```python
from build123d import *

# Parameters (mm, degrees)
SKETCH4_W                      = 116
SKETCH4_H                      = 116
BOSS_EXTRUDE1_DEPTH            = 10
SKETCH6_R                      = 33.5
CUT_EXTRUDE1_DEPTH             = 83.63171304
BOSS_EXTRUDE3_DEPTH            = 8.4
SKETCH10_W                     = 116
SKETCH10_H                     = 116
BOSS_EXTRUDE5_DEPTH            = 15
SKETCH11_R                     = 4
POSITIONING_HOLE_DEPTH         = 28
SKETCH23_R                     = 4
SNAPPING_HOLE_DEPTH            = 28
SKETCH13_R                     = 34.75
SKETCH13_R_2                   = 33.5
BOSS_EXTRUDE6_DEPTH            = 25
SKETCH24_W                     = 40
SKETCH24_H                     = 8
BOSS_EXTRUDE7_DEPTH            = 150
BOSS_EXTRUDE9_DEPTH            = 40
CUT_EXTRUDE6_DEPTH             = 8
CUT_EXTRUDE6_DIRECTION_2_REACH = 229.876
CUT_EXTRUDE7_REACH             = 225.194
CUT_EXTRUDE9_REACH             = 209.566
SKETCH37_W                     = 25
SKETCH37_H                     = 20
SKETCH12_R                     = 33.5
MAIN_HOLE_DEPTH                = 179.740034687
SKETCH42_R                     = 54
SKETCH42_R_2                   = 51
BOSS_EXTRUDE12_DEPTH           = 150
CHAMFER3_SIZE                  = 5
SKETCH44_W                     = 40.182717611
SKETCH44_H                     = 23
BOSS_EXTRUDE15_DEPTH           = 150
SKETCH41_R                     = 2
BOSS_EXTRUDE11_DEPTH           = 5
CUT_EXTRUDE12_START            = -150
SKETCH45_R                     = 51
CUT_EXTRUDE12_DEPTH            = 150
SKETCH46_R                     = 1
CUT_EXTRUDE13_DEPTH            = 25


with BuildPart() as part:
    # Sketch4 → Boss-Extrude1 (new body)
    with BuildSketch(Plane(origin=(0, 0, 0), x_dir=(1, 0, 0), z_dir=(0, 1, 0))):
        Rectangle(SKETCH4_W, SKETCH4_H)
    extrude(amount=BOSS_EXTRUDE1_DEPTH)

    # Sketch6 → Cut-Extrude1 (cut, through all)
    with BuildSketch(Plane(origin=(0, 10, 0), x_dir=(1, 0, 0), z_dir=(0, 1, 0))):
        with Locations(Location((0, 0, 0), (0, 0, 270))):
            Circle(SKETCH6_R)
    extrude(amount=-CUT_EXTRUDE1_DEPTH, mode=Mode.SUBTRACT)

    # Sketch8 → Boss-Extrude3 (add)
    with BuildSketch(Plane.XZ):
        with BuildLine():
            Line((-58, 58), (-58, -58))
            Line((-58, -58), (22, -58))
            ThreePointArc((22, -58), (-36, 0), (22, 58))
            Line((22, 58), (-58, 58))
        make_face()
    extrude(amount=BOSS_EXTRUDE3_DEPTH)

    # Sketch10 → Boss-Extrude5 (add)
    with BuildSketch(Plane.XZ.offset(8.4)):
        Rectangle(SKETCH10_W, SKETCH10_H)
    extrude(amount=BOSS_EXTRUDE5_DEPTH)

    # Sketch11 → positioning hole (cut)
    with BuildSketch(Plane.XZ.offset(23.4)):
        with Locations(Location((39, 0, 0), (0, 0, 270))):
            Circle(SKETCH11_R)
    extrude(amount=-POSITIONING_HOLE_DEPTH, mode=Mode.SUBTRACT)

    # Sketch23 → snapping hole (cut)
    with BuildSketch(Plane.XZ.offset(23.4)):
        with Locations(Location((38.947036647, 20, 0), (0, 0, 270))):
            Circle(SKETCH23_R)
    extrude(amount=-SNAPPING_HOLE_DEPTH, mode=Mode.SUBTRACT)

    # Sketch13 → Boss-Extrude6 (add)
    with BuildSketch(Plane.XZ.offset(23.4)):
        with Locations(Location((0, 0, 0), (0, 0, 270))):
            Circle(SKETCH13_R)
        with Locations(Location((0, 0, 0), (0, 0, 90))):
            Circle(SKETCH13_R_2, mode=Mode.SUBTRACT)
    extrude(amount=BOSS_EXTRUDE6_DEPTH)

    # Sketch24 → Boss-Extrude7 (add)
    with BuildSketch(Plane.XZ.offset(23.4)):
        with Locations((0, 54)):
            Rectangle(SKETCH24_W, SKETCH24_H)
        with Locations((0, -54)):
            Rectangle(SKETCH24_W, SKETCH24_H)
    extrude(amount=BOSS_EXTRUDE7_DEPTH)

    # Sketch28 → Boss-Extrude9 (add)
    with BuildSketch(Plane.ZY.offset(20)):
        Polygon((-58, -173.4), (-58, 10), (-78, 10), align=None)
        Polygon((58, 10), (58, -173.4), (78, 10), align=None)
    extrude(amount=-BOSS_EXTRUDE9_DEPTH)

    # Sketch31 → Cut-Extrude6 (cut)
    with BuildSketch(Plane(origin=(0, 0, -58), x_dir=(-1, 0, 0), z_dir=(0, 0, -1))):
        with BuildLine():
            Line((2.5, -28.4), (2.5, -168.4))
            ThreePointArc((2.5, -168.4), (0, -170.9), (-2.5, -168.4))
            Line((-2.5, -168.4), (-2.5, -28.4))
            ThreePointArc((-2.5, -28.4), (0, -25.9), (2.5, -28.4))
        make_face()
    extrude(amount=-CUT_EXTRUDE6_DEPTH, mode=Mode.SUBTRACT)

    # Cut-Extrude6 direction 2: up to this plane
    cut_extrude6_direction_2_end = Plane(origin=(20, 10, -78), z_dir=(0, -0.1084085524287415, -0.9941064257715594))
    # Sketch31 → Cut-Extrude6 direction 2 (cut, up to the surface)
    with BuildSketch(Plane(origin=(0, 0, -58), x_dir=(-1, 0, 0), z_dir=(0, 0, -1)), mode=Mode.PRIVATE) as cut_extrude6_direction_2_sk1:
        with BuildLine():
            Line((2.5, -28.4), (2.5, -168.4))
            ThreePointArc((2.5, -168.4), (0, -170.9), (-2.5, -168.4))
            Line((-2.5, -168.4), (-2.5, -28.4))
            ThreePointArc((-2.5, -28.4), (0, -25.9), (2.5, -28.4))
        make_face()
    cut_extrude6_direction_2_tool1 = split(extrude(cut_extrude6_direction_2_sk1.sketch, amount=CUT_EXTRUDE6_DIRECTION_2_REACH, mode=Mode.PRIVATE), bisect_by=cut_extrude6_direction_2_end, keep=Keep.BOTH, mode=Mode.PRIVATE)
    add(cut_extrude6_direction_2_tool1.solids().sort_by_distance((0, -98.4, -58))[0], mode=Mode.SUBTRACT)

    # Cut-Extrude7: up to this plane
    cut_extrude7_end = Plane(origin=(20, -173.4, 58), z_dir=(0, -0.1084085524287415, 0.9941064257715594))
    # Sketch34 → Cut-Extrude7 (cut, up to the surface)
    with BuildSketch(Plane(origin=(0, 0, 50), x_dir=(-1, 0, 0), z_dir=(0, 0, -1)), mode=Mode.PRIVATE) as cut_extrude7_sk1:
        with BuildLine():
            Line((-2.5, -28.4), (-2.5, -168.4))
            ThreePointArc((-2.5, -168.4), (0, -170.9), (2.5, -168.4))
            Line((2.5, -168.4), (2.5, -28.4))
            ThreePointArc((2.5, -28.4), (0, -25.9), (-2.5, -28.4))
        make_face()
    cut_extrude7_tool1 = split(extrude(cut_extrude7_sk1.sketch, amount=-CUT_EXTRUDE7_REACH, mode=Mode.PRIVATE), bisect_by=cut_extrude7_end, keep=Keep.BOTH, mode=Mode.PRIVATE)
    add(cut_extrude7_tool1.solids().sort_by_distance((0, -98.4, 50))[0], mode=Mode.SUBTRACT)

    # Sketch37 → Cut-Extrude9 (cut, up to next)
    with BuildSketch(Plane(origin=(0, 10, 0), x_dir=(1, 0, 0), z_dir=(0, 1, 0)), mode=Mode.PRIVATE) as cut_extrude9_sk1:
        with Locations((0, 68)):
            Rectangle(SKETCH37_W, SKETCH37_H)
    cut_extrude9_tool1 = extrude(cut_extrude9_sk1.sketch, amount=-CUT_EXTRUDE9_REACH, mode=Mode.PRIVATE) & part.part
    # Sketch37 → Cut-Extrude9 (cut, up to next)
    with BuildSketch(Plane(origin=(0, 10, 0), x_dir=(1, 0, 0), z_dir=(0, 1, 0)), mode=Mode.PRIVATE) as cut_extrude9_sk2:
        with Locations((0, -68)):
            Rectangle(SKETCH37_W, SKETCH37_H)
    cut_extrude9_tool2 = extrude(cut_extrude9_sk2.sketch, amount=-CUT_EXTRUDE9_REACH, mode=Mode.PRIVATE) & part.part
    add(cut_extrude9_tool1.solids().sort_by_distance((0, 10, -68))[0], mode=Mode.SUBTRACT)
    add(cut_extrude9_tool2.solids().sort_by_distance((0, 10, 68))[0], mode=Mode.SUBTRACT)

    # Sketch12 → main hole (cut, through all)
    with BuildSketch(Plane.XZ.offset(23.4)):
        with Locations(Location((0, 0, 0), (0, 0, 90))):
            Circle(SKETCH12_R)
    extrude(amount=-MAIN_HOLE_DEPTH, mode=Mode.SUBTRACT)

    # Sketch42 → Boss-Extrude12 (add)
    with BuildSketch(Plane(origin=(0, 10, 0), x_dir=(1, 0, 0), z_dir=(0, 1, 0))):
        with Locations(Location((0, 0, 0), (0, 0, 270))):
            Circle(SKETCH42_R)
        with Locations(Location((0, 0, 0), (0, 0, 270))):
            Circle(SKETCH42_R_2, mode=Mode.SUBTRACT)
    extrude(amount=BOSS_EXTRUDE12_DEPTH)

    # Chamfer3
    chamfer3_edges = [part.edges().sort_by_distance(p)[0] for p in [
        (0, 10, -33.5),
    ]]
    chamfer(chamfer3_edges, length=CHAMFER3_SIZE)

    # Sketch44 → Boss-Extrude15 (add)
    with BuildSketch(Plane(origin=(0, 10, 0), x_dir=(1, 0, 0), z_dir=(0, 1, 0))):
        with Locations((0.091358806, 66.5)):
            Rectangle(SKETCH44_W, SKETCH44_H)
        with Locations((0.091358806, -66.5)):
            Rectangle(SKETCH44_W, SKETCH44_H)
    extrude(amount=BOSS_EXTRUDE15_DEPTH)

    # Sketch41 → Boss-Extrude11 (add)
    with BuildSketch(Plane(origin=(0, 160, 0), x_dir=(1, 0, 0), z_dir=(0, 1, 0))):
        Polygon((45, 105), (105, 105), (105, -105), (-105, -105), (-105, 105), (-45, 105), (-45, 130), (45, 130), align=None)
        with Locations(Location((-100, -100, 0), (0, 0, 270))):
            Circle(SKETCH41_R, mode=Mode.SUBTRACT)
        with Locations(Location((100, -100, 0), (0, 0, 270))):
            Circle(SKETCH41_R, mode=Mode.SUBTRACT)
    extrude(amount=BOSS_EXTRUDE11_DEPTH)

    # Sketch45 → Cut-Extrude12 (cut)
    with BuildSketch(Plane(origin=(0, 165, 0), x_dir=(1, 0, 0), z_dir=(0, 1, 0)).offset(CUT_EXTRUDE12_START)):
        with Locations(Location((0, 0, 0), (0, 0, 270))):
            Circle(SKETCH45_R)
    extrude(amount=CUT_EXTRUDE12_DEPTH, mode=Mode.SUBTRACT)

    # Sketch46 → Cut-Extrude13 (cut)
    with BuildSketch(Plane(origin=(20, 0, 0), x_dir=(0, 0, -1), z_dir=(1, 0, 0))):
        with Locations((-73.540080926, 6)):
            Circle(SKETCH46_R)
        with Locations((-73.10387591, 2)):
            Circle(SKETCH46_R)
    extrude(amount=-CUT_EXTRUDE13_DEPTH, mode=Mode.SUBTRACT)


solid = part.part
```
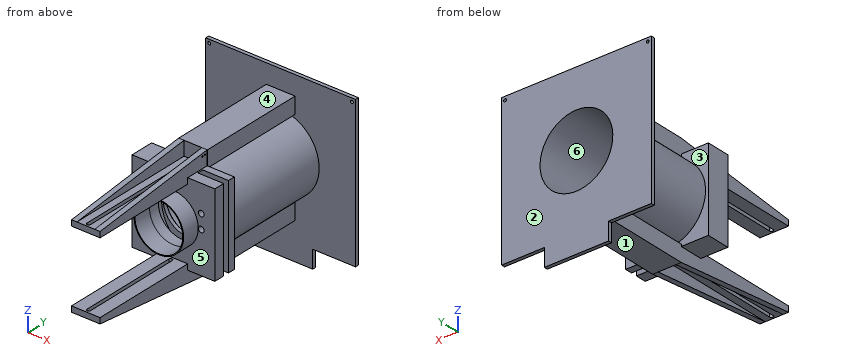
Source: CAD feature listing. Evaluate the final solid. Frame: model axes, mm. Face numbers are marked on the shaded views. A direction names the side the tool comes from. Coordinates: 2 decimals unless noted, no trailing zeros. Loops run counter-clockwise (first coordinate to the right, second up) from the corner with the lowest first, then second, coordinate; pieces in that order, holes last. Notation, with made-up numbers: (-31.75, -11) - (20.25, -11) arc R7 ccw to (20.25, -4) - close; hole circle Ø6 at (-14.5, 8.25). An arc over 180 degrees is marked (long way). Answer as CSV lines item,"result".
1. Reachability of the marked faces 4, 5 and 6 from +Z, -Z, +X, -X, +Y, -Y: full face, straight path, thin tool, end or side. Return the list, or none.
Established:
face 4,"+Z, +X, -X, -Y"
face 5,"-Y"
face 6,"+Y"
2. Mould query, pull axis Y, two halves, no side actions, for the marked faces 1, 2 and 3. Classes: released by +Y, released by -Y, zero draft, split by the parting line, or undercut.
Established:
face 1,"zero draft"
face 2,"released by +Y"
face 3,"undercut"
3. Section C-C (y = -19.5). Return loops of the section in (x, z), then the cut area to 3 significant figures.
Established:
outline,"(-58, -58) - (-20, -58) - (-20, -74.78) - (-12.5, -74.78) - (-12.5, -58) - (12.5, -58) - (12.5, -74.78) - (20, -74.78) - (20, -58) - (58, -58) - (58, 58) - (20, 58) - (20, 74.78) - (12.5, 74.78) - (12.5, 58) - (-12.5, 58) - (-12.5, 74.78) - (-20, 74.78) - (-20, 58) - (-58, 58) - close; hole circle Ø67 at (0, 0); hole circle Ø8 at (38.95, 20); hole circle Ø8 at (39, 0)"
area,"10,300 mm2"
4. Ray query, line 1 (Z direction, x = 2.5, y = 53.5); line 2 (Y direction, x = 53.5, z = -31); line 3 (X direction, y = -18, z = 0). Return the intervals inside material, ascending.
Established:
line 1,"z = -78 to -55, -53.94 to -50.94, 50.94 to 53.94, 55 to 78"
line 2,"y = -23.4 to -8.4, 0 to 10, 160 to 165"
line 3,"x = -58 to -33.5, 33.5 to 35, 43 to 58"
5. Section B-B (z = 0). Count the separate pieces of the cut face and the enclosed holes in it, then the cut area to 3 significant figures.
Established:
separate pieces,"4"
enclosed holes,"0"
area,"2,730 mm2"
6. Section A-A (y = 131.5). Return loops of the section in (x, z).
Established:
outline,"circle Ø108 at (0, 0); (-20, -78) - (20.18, -78) - (20.18, -55) - (-20, -55) - close; (-20, 55) - (20.18, 55) - (20.18, 78) - (-20, 78) - close; hole circle Ø102 at (0, 0)"
7. Contact query for flat-ended pins moving along their axis: pin 1 (4 mm diameter, centred on y = 163, z = -118, fed in from -X); pin 2 (10 mm diameter, centred on y = 41, z = 46.5, fed in from -X); pin 3 (1.8 mm diameter, centred on y = 2, z = 73.1, fed in from +X). Output: stop coordinate, or through.
Established:
pin 1,"stops at x = -45"
pin 2,"stops at x = -34.55"
pin 3,"stops at x = -12.5"
